```python
from build123d import *

# Parameters (mm, degrees)
EXTRUDE_THIN1_DEPTH        = 101.6
EXTRUDE_THIN1_DEPTH_BACK   = 6.35
EXTRUDE_THIN1_2_DEPTH      = 101.6
EXTRUDE_THIN1_2_DEPTH_BACK = 6.35
BOSS_EXTRUDE1_DEPTH        = 6.35
SKETCH2_W                  = 25.4
SKETCH2_H                  = 50.8
BOSS_EXTRUDE2_DEPTH        = 50.8
SKETCH3_R                  = 14.2875
CUT_EXTRUDE1_DEPTH         = 496.3
SKETCH4_W                  = 495.3
SKETCH4_H                  = 6.35
BOSS_EXTRUDE3_DEPTH        = 139.7


with BuildPart() as part:
    # Sketch1 → Extrude-Thin1 (new body, two sides)
    with BuildSketch(Plane.XY) as extrude_thin1_sk:
        Polygon((0, 0), (0, 76.2), (177.8, 441.642362076), (177.8, 517.842362076), (184.15, 517.842362076), (184.15, 440.179589293), (6.35, 74.737227217), (6.35, 0), align=None)
    extrude(amount=EXTRUDE_THIN1_DEPTH)
    extrude(extrude_thin1_sk.sketch, amount=-EXTRUDE_THIN1_DEPTH_BACK)



with BuildPart() as body_2:
    # Sketch1 → Extrude-Thin1 2 (new body, two sides)
    with BuildSketch(Plane.XY) as extrude_thin1_2_sk:
        Polygon((-304.8, 517.842362076), (-304.8, 441.642362076), (-127, 76.2), (-127, 0), (-133.35, 0), (-133.35, 74.737227217), (-311.15, 440.179589293), (-311.15, 517.842362076), align=None)
    extrude(amount=EXTRUDE_THIN1_2_DEPTH)
    extrude(extrude_thin1_2_sk.sketch, amount=-EXTRUDE_THIN1_2_DEPTH_BACK)

    # Sketch1<3> → Boss-Extrude1 (add)
    with BuildSketch(Plane.XY):
        Polygon((-127, 0), (0, 0), (0, 76.2), (177.8, 441.642362076), (177.8, 517.842362076), (-304.8, 517.842362076), (-304.8, 441.642362076), (-127, 76.2), align=None)
    extrude(amount=-BOSS_EXTRUDE1_DEPTH)


with BuildPart() as part_1:
    add(part.part)

    add(body_2.part)  # Boss-Extrude2 merges body 2
    # Sketch2 → Boss-Extrude2 (add)
    with BuildSketch(Plane(origin=(0, 0, -6.35), x_dir=(-1, 0, 0), z_dir=(0, 0, -1))):
        with Locations((-171.45, 492.442362076)):
            Rectangle(SKETCH2_W, SKETCH2_H)
        with Locations((298.45, 492.442362076)):
            Rectangle(SKETCH2_W, SKETCH2_H)
    extrude(amount=BOSS_EXTRUDE2_DEPTH)

    # Sketch3 → Cut-Extrude1 (cut, through all)
    with BuildSketch(Plane(origin=(184.15, 0, 0), x_dir=(0, 0, -1), z_dir=(1, 0, 0))):
        with Locations((31.75, 492.442362076)):
            Circle(SKETCH3_R)
    extrude(amount=-CUT_EXTRUDE1_DEPTH, mode=Mode.SUBTRACT)

    # Sketch4 → Boss-Extrude3 (add)
    with BuildSketch(Plane(origin=(0, 517.842362076, 0), x_dir=(1, 0, 0), z_dir=(0, 1, 0))):
        with Locations((-63.5, 3.175)):
            Rectangle(SKETCH4_W, SKETCH4_H)
    extrude(amount=BOSS_EXTRUDE3_DEPTH)


solid = part_1.part
```
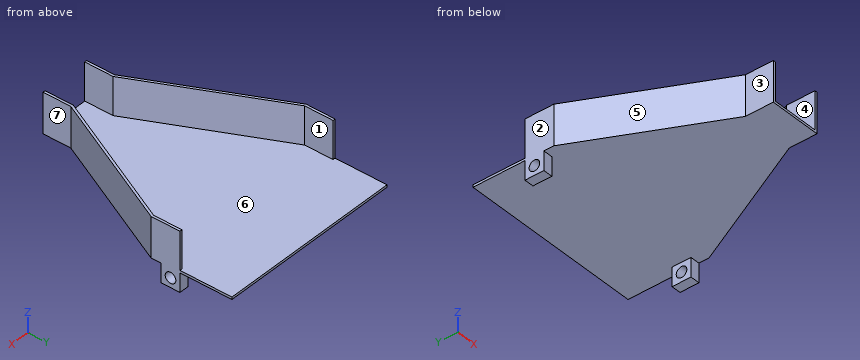
Geometry check sheet. Reference: the model listing, model coordinates, mm. Face numbers are marked on the shaded views. A direction names the side the tool comes from. Coordinates: 2 decimals unless noted, no trailing zeros. Order: outer loops, then holes, each group sorted by start corner. A loop starts at its lowest first (then second) coordinate and runs counter-clockwise, first axis right, second up.
Q1. Depth check by flat-ended pin: pin 1 Ø12 at (y, z) = (526, 48) entering from -X; pin 2 Ø22.5 at (y, z) = (53, 64) entering from -X; pin 3 Ø6 at (y, z) = (368, 14) entering from +X; pin 4 Ø1 at (x, z) = (25, 66) entering from +Y. Enter the tip coordinate at first touch or a pass-through.
Reply:
pin 1: passes through
pin 2: stops at x = -133.35
pin 3: stops at x = 150.49
pin 4: stops at y = 128.61
Q2. Sectioned sample at B-B on z = -31.75. Record the cut outline in (x, y).
Reply:
outline: (-311.15, 467.04) - (-285.75, 467.04) - (-285.75, 478.15) - (-311.15, 478.15) - close; (-311.15, 506.73) - (-285.75, 506.73) - (-285.75, 517.84) - (-311.15, 517.84) - close; (158.75, 467.04) - (184.15, 467.04) - (184.15, 478.15) - (158.75, 478.15) - close; (158.75, 506.73) - (184.15, 506.73) - (184.15, 517.84) - (158.75, 517.84) - close
Q3. Tool access check on the marked faces 1, 2, 3 and 4. Record the directions out of +Z, -Z, +X, -X, +Y, -Y that give a thin tool (end or side, any length) a straight path to the whole face; none if there is none.
Reply:
face 1: +Z, +Y
face 2: +Z, -Z, -X, +Y, -Y
face 3: +Z, -Z, -X, -Y
face 4: +Z, +Y, -Y
Q4. Draft check along X on the marked faces 5, 6 and 7. Enter one of: released by +X, released by -X, zero draft, split by the parting line, or undercut.
Reply:
face 5: released by -X
face 6: undercut
face 7: released by +X
Q5. Sectioned sample at D-D on x = -39. Record the cut outline in (y, z).
Reply:
outline: (0, -6.35) - (657.54, -6.35) - (657.54, 0) - (0, 0) - close
Q6. Sectioned sample at C-C on y = 268. Record the cut outline in (x, z).
Reply:
outline: (-227.38, -6.35) - (100.38, -6.35) - (100.38, 101.6) - (93.32, 101.6) - (93.32, 0) - (-220.32, 0) - (-220.32, 101.6) - (-227.38, 101.6) - close
Q7. Thickness scan on probe 1 along X at (y, z) = (507, 56); probe 2 along Y at (x, z) = (-300, -31); probe 3 along Z at (x, y) = (-99, 271.5). Record the ranges inside material, lowest first.
Reply:
probe 1: x = -311.15 to -304.8, 177.8 to 184.15
probe 2: y = 467.04 to 478.17, 506.71 to 517.84
probe 3: z = -6.35 to 0
Q8. Sectioned sample at A-A on z = 38. Record the cut outline in (x, y).
Reply:
outline: (-311.15, 440.18) - (-133.35, 74.74) - (-133.35, 0) - (-127, 0) - (-127, 76.2) - (-304.8, 441.64) - (-304.8, 517.84) - (-311.15, 517.84) - close; (0, 0) - (6.35, 0) - (6.35, 74.74) - (184.15, 440.18) - (184.15, 517.84) - (177.8, 517.84) - (177.8, 441.64) - (0, 76.2) - close
